Part print with two shaded views. Sizes in mm from the minimum x, y, z corner. Round coordinates to 2 decimals unless told otherwise and drop trailing zeros. Order: outer loops, then holes, each group sorted by start corner. A loop starts at its lowest first (then second) coordinate and runs counter-clockwise, first axis right, second up. Notation, with made-up numbers: M -14,3.25 L 19,3.25 A28 cw 19,41.25 Z; hole C -32.75,65 d2. An arc over 180 degrees is marked long. One line per question, with ' | ' between items. Start each with the question number.
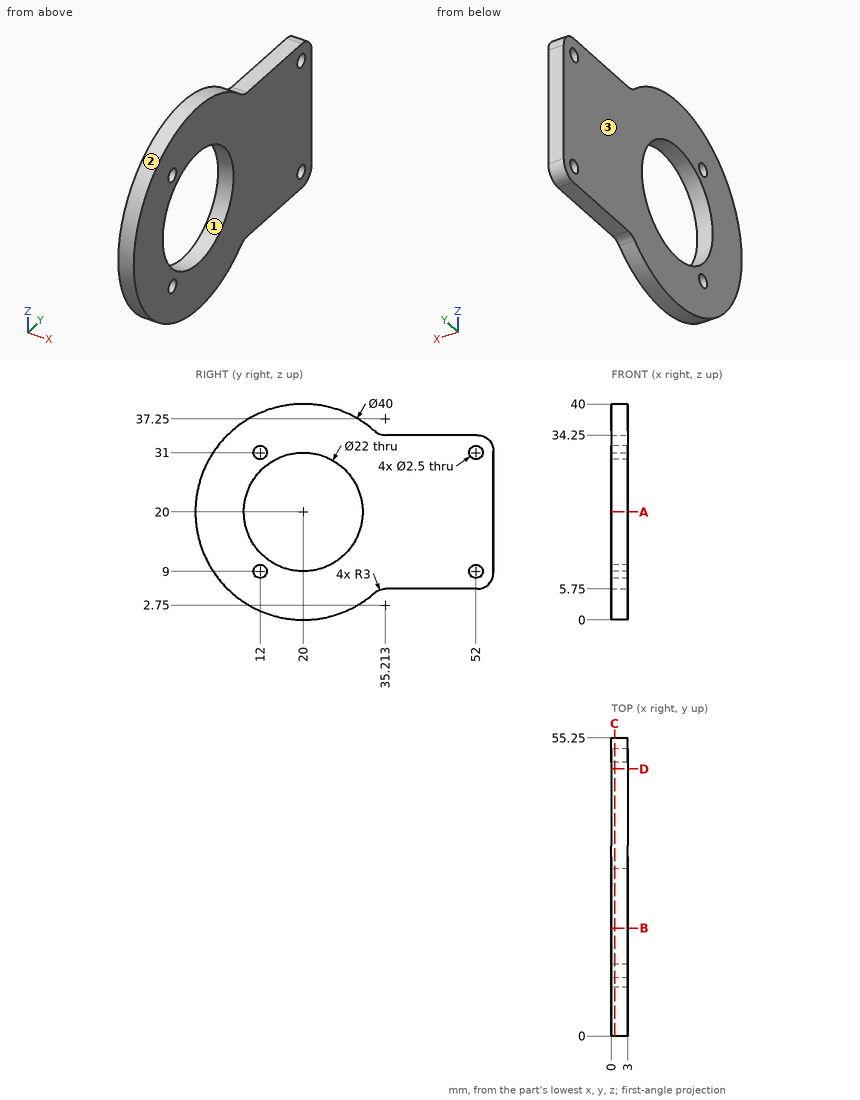
Item 1: Cut at A-A on z = 20. Write the cut outline in (x, y).
Item 2: Cut at D-D on y = 49.5. Write the cut outline in (x, z), then the cut area to 3 significant figures.
Item 3: Flat gauge pins, fed straight in: pin 1 (1.5 mm diameter, centred on y = 12, z = 31, fed in from -X); pin 2 (1.5 mm diameter, centred on x = 1.5, y = 42, fed in from -Z); pin 3 (1.5 mm diameter, centred on x = 2, y = 41.5, fed in from +Z). Where does each tip first touch, or does it go through?
Item 4: Wall check: line 1 along Z through (x, y) = (1.2, 52); line 2 along Z through (x, y) = (0.65, 12); line 3 along Z through (x, y) = (2.3, 38). Give the ranges that are in metal, low to high. Write a range as [from, to].
Item 5: Cut at B-B on y = 20. Write the cut outline in (x, z), then the cut area to 3 significant figures.
Item 6: Cut at C-C on x = 0.6. Write the cut outline in (y, z), then the cut area to 3 significant figures.
Item 7: Two-plate mould, pull along Z, no slides. Class the marked faces 1, 2 and 3: +Z half, -Z half, draft (parallel to the pull), parting line (faces both ways), or undercut.
Results found:
1) outline: M 0,0 L 3,0 L 3,9 L 0,9 Z; M 0,31 L 3,31 L 3,55.25 L 0,55.25 Z
2) outline: M 0,5.75 L 3,5.75 L 3,34.25 L 0,34.25 Z | area: 85.5 mm^2
3) pin 1: passes through | pin 2: stops at z = 5.75 | pin 3: stops at z = 34.25
4) line 1: z = [5.75, 7.75], [10.25, 29.75], [32.25, 34.25] | line 2: z = [1.67, 7.75], [10.25, 12.45], [27.55, 29.75], [32.25, 38.33] | line 3: z = [5.75, 34.25]
5) outline: M 0,0 L 3,0 L 3,9 L 0,9 Z; M 0,31 L 3,31 L 3,40 L 0,40 Z | area: 54.0 mm^2
6) outline: M 33.23,5 A3 cw 35.21,5.75 L 52.25,5.75 A3 ccw 55.25,8.75 L 55.25,31.25 A3 ccw 52.25,34.25 L 35.21,34.25 A3 cw 33.23,35 A20 ccw long Z; hole C 20,20 d22; hole C 12,9 d2.5; hole C 12,31 d2.5; hole C 52,9 d2.5; hole C 52,31 d2.5 | area: 1,340 mm^2
7) face 1: undercut | face 2: parting line | face 3: draft
